Autodesk Inventor part; units mm, degrees
ref_plane "YZ Plane" through (0, 0, 0) normal (1, 0, 0) x (0, 1, 0)
ref_plane "XZ Plane" through (0, 0, 0) normal (0, 1, 0) x (-1, 0, 0)
ref_plane "XY Plane" through (0, 0, 0) normal (0, 0, 1) x (1, 0, 0)
sketch "Sketch1" plane through (0, 0, 0) normal (0, 1, 0) x (-1, 0, 0)
  line L0 (2.375, 7.35) -> (-2.375, 7.35)
  line L1 (-2.375, 7.35) -> (-2.375, -7.35)
  line L2 (-2.375, -7.35) -> (2.375, -7.35)
  line L3 (2.375, -7.35) -> (2.375, 7.35)
  point P0 (0, 0)
  dimension "d0" = 14.7
  dimension "d1" = 4.75
  dimension "d2" = 2.375
  dimension "d3" = 7.35
extrude "Extrusion1" add sketch "Sketch1" along normal blind 3.2
sketch "Sketch2" plane through (0, 0, 0) normal (0, -1, 0) x (1, 0, 0)
  circle A0 centre (0, 5.895) radius 0.5
  circle A1 centre (0, 2.235) radius 0.5
  point P0 (0, 0)
  dimension "d6" = 3.66
  dimension "d7" = 2.235
  dimension "d8" = 1
  dimension "d9" = 1
extrude "Extrusion2" add sketch "Sketch2" along normal blind 2.3
sketch "Sketch3" plane through (0, 3.2, 0) normal (0, 1, 0) x (1, 0, 0)
  line L0 (-1, -5.98) -> (1, -5.98)
  line L1 (1, -5.98) -> (1, -2.02)
  line L2 (1, -2.02) -> (-1, -2.02)
  line L3 (-1, -2.02) -> (-1, -5.98)
  line L4 (-1, -4) -> (1, -4) construction
  line L5 (-0.6, -5.45) -> (0.4, -5.45)
  line L6 (0.4, -5.45) -> (0.4, -2.4349)
  line L7 (0.4, -2.4349) -> (-0.6, -2.4349)
  line L8 (-0.6, -2.4349) -> (-0.6, -5.45)
  line L9 (0.4, -4.5) -> (1, -4.5)
  line L10 (1, -4.5) -> (1, -3.5)
  line L11 (1, -3.5) -> (0.4, -3.5)
  line L12 (0.4, -3.5) -> (0.4, -4.5)
  point P0 (0, 0)
  dimension "d12" = 4
  dimension "d13" = 3.96
  dimension "d14" = 1
  dimension "d15" = 0.4
  dimension "d16" = 5.45
  dimension "d17" = 3.0151
  dimension "d18" = 2
  dimension "d19" = 1
  dimension "d20" = 0.5
  dimension "d21" = 1
extrude "Extrusion3" add sketch "Sketch3" along normal blind 5 contours L3 L2 L1 L11 L6 L7 L8 L5 L9 L0
mirror "Mirror1" about plane through (0, 0, 0) normal (0, 0, 1) of "Extrusion3", "Extrusion2"
properties part number "BK-6013_MiniATC_Fuse_Holder"
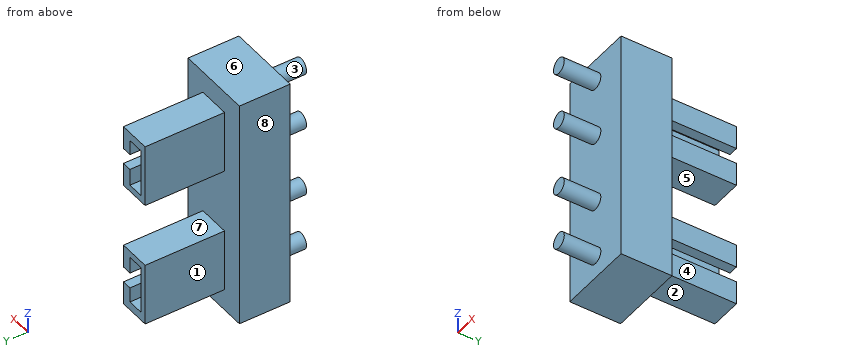
Design review of the part built by this model. Coordinates are the model's own, in mm. Face numbers are marked on the shaded views. A direction names the side the tool comes from. Coordinates: 2 decimals unless noted, no trailing zeros. Loops run counter-clockwise (first coordinate to the right, second up) from the corner with the lowest first, then second, coordinate; pieces in that order, holes last. Notation, with made-up numbers: (79.5, 10) -> (124.5, 10) arc R28 cw to (124.5, 28) -> close; hole circle Ø6 at (76.5, 23). An arc over 180 degrees is marked (long way). Answer as a JSON object with one key per item and string values.
Q1. Tool access review of the marked faces 1, 2, 3, 4 and 5: name each direction out of +Z, -Z, +X, -X, +Y, -Y from which nothing blocks a thin tool from reaching the whole face with its end or side.
Answer block:
{"face 1": "+Z, -Z, -X, +Y", "face 2": "-Z, +X, -X, +Y", "face 3": "-Y", "face 4": "+Z, -Z, +X, +Y", "face 5": "+X, -X, +Y"}
Q2. Take a section at D-D on y = -1. Give the boundary of the cut face in (x, z) (3 decimals), plus the area to 3 significant figures.
Answer block:
{"outline": "circle Ø1 at (0, -5.895); circle Ø1 at (0, -2.235); circle Ø1 at (0, 2.235); circle Ø1 at (0, 5.895)", "area": "3.14 mm^2"}
Q3. Take a section at A-A on y = 3.5. Give the boundary of the cut face in (x, z), plus the area to 3 significant figures.
Answer block:
{"outline": "(-1, -5.98) -> (1, -5.98) -> (1, -4.5) -> (0.4, -4.5) -> (0.4, -5.45) -> (-0.6, -5.45) -> (-0.6, -2.43) -> (0.4, -2.43) -> (0.4, -3.5) -> (1, -3.5) -> (1, -2.02) -> (-1, -2.02) -> close; (-1, 2.02) -> (1, 2.02) -> (1, 3.5) -> (0.4, 3.5) -> (0.4, 2.43) -> (-0.6, 2.43) -> (-0.6, 5.45) -> (0.4, 5.45) -> (0.4, 4.5) -> (1, 4.5) -> (1, 5.98) -> (-1, 5.98) -> close", "area": "8.61 mm^2"}
Q4. To check wall thickness, follow L1, parallel to Z at x = 0.5, y = 5.25; L2, parallel to X at y = 5.5, z = 5.25; L3, parallel to Y at x = 0.9, z = 2.5. State the ranges of each line that lie inside material, in increasing order.
Answer block:
{"L1": "z = -5.98 to -4.5, -3.5 to -2.02, 2.02 to 3.5, 4.5 to 5.98", "L2": "x = -1 to -0.6, 0.4 to 1", "L3": "y = 0 to 8.2"}
Q5. Take a section at C-C on z = 4. Give the boundary of the cut face in (x, y) (3 decimals), plus the area to 3 significant figures.
Answer block:
{"outline": "(-2.375, 0) -> (2.375, 0) -> (2.375, 3.2) -> (-0.6, 3.2) -> (-0.6, 8.2) -> (-1, 8.2) -> (-1, 3.2) -> (-2.375, 3.2) -> close", "area": "17.2 mm^2"}
Q6. Take a section at B-B on x = 0.7. Give the boundary of the cut face in (y, z).
Answer block:
{"outline": "(0, -7.35) -> (3.2, -7.35) -> (3.2, -5.98) -> (8.2, -5.98) -> (8.2, -4.5) -> (3.2, -4.5) -> (3.2, -3.5) -> (8.2, -3.5) -> (8.2, -2.02) -> (3.2, -2.02) -> (3.2, 2.02) -> (8.2, 2.02) -> (8.2, 3.5) -> (3.2, 3.5) -> (3.2, 4.5) -> (8.2, 4.5) -> (8.2, 5.98) -> (3.2, 5.98) -> (3.2, 7.35) -> (0, 7.35) -> close"}
Q7. The part is to be moulded in two halves that separate along Z. For the marked faces 6, 7 and 8, say which applies: +Z half, -Z half, draft (parallel to the pull), parting line (faces both ways), or undercut.
Answer block:
{"face 6": "+Z half", "face 7": "undercut", "face 8": "draft"}
Q8. Clearance check with flat-ended pins moving along their axes: pin 1 Ø1 at (x, y) = (-0.5, 6) entering from -Z; pin 2 Ø1.4 at (x, z) = (-1, -1) entering from +Y; pin 3 Ø0.5 at (y, z) = (6.5, 3) entering from -X. State where each tip first meets the part, or that it passes through.
Answer block:
{"pin 1": "stops at z = -5.98", "pin 2": "stops at y = 3.2", "pin 3": "stops at x = -1"}
